from build123d import *

# Parameters (mm, degrees)
F1_W           = 102
F1_H           = 42
F1_W_2         = 98
F1_H_2         = 38
F2_DEPTH       = 72
F3_R           = 8.1966630734
F4_DEPTH       = 25
F6_D           = 3.1
F6_DEPTH       = 20
F6_CSINK_D     = 5.5
F6_CSINK_ANGLE = 90
F6_TIP         = 0.9313339595
F7_W           = 102
F7_H           = 42
F8_DEPTH       = 2
F10_D          = 4
F10_DEPTH      = 20
F10_TIP        = 1.2017212381


with BuildPart() as f2:
    # F1 (on Top) → F2 (new body)
    with BuildSketch(Plane.XY):
        Rectangle(F1_W, F1_H)
        Rectangle(F1_W_2, F1_H_2, mode=Mode.SUBTRACT)
    extrude(amount=F2_DEPTH)

    # F3 (on face) → F4 (cut)
    with BuildSketch(Plane(origin=(0, 0, 0), x_dir=(1, 0, 0), z_dir=(0, 0, -1))):
        Circle(F3_R)
    extrude(amount=-F4_DEPTH, mode=Mode.SUBTRACT)

    # F6
    with Locations(Plane(origin=(-51, 0, 0), x_dir=(0, -1, 0), z_dir=(-1, 0, 0))):
        with Locations((0, 67)):
            CounterSinkHole(F6_D / 2, F6_CSINK_D / 2, depth=F6_DEPTH, counter_sink_angle=F6_CSINK_ANGLE)
            with Locations((0, 0, -(F6_DEPTH + F6_TIP / 2))):  # 118° drill point
                Cone(0, F6_D / 2, F6_TIP, mode=Mode.SUBTRACT)

    # F7 (on Top) → F8 (join)
    with BuildSketch(Plane.XY):
        Rectangle(F7_W, F7_H)
    extrude(amount=F8_DEPTH)

    # F10
    with Locations(Plane(origin=(0, 0, 0), x_dir=(1, 0, 0), z_dir=(0, 0, -1))):
        with Locations((25.5, 10.5), (-25.5, 10.5)):
            Hole(F10_D / 2, depth=F10_DEPTH)
            with Locations((0, 0, -(F10_DEPTH + F10_TIP / 2))):  # 118° drill point
                Cone(0, F10_D / 2, F10_TIP, mode=Mode.SUBTRACT)


solid = f2.part
CAD build for the part. Positions are in the model's coordinates, mm. A direction names the side the tool comes from. Coordinates: 2 decimals unless noted, no trailing zeros. Loops run counter-clockwise (first coordinate to the right, second up) from the corner with the lowest first, then second, coordinate; pieces in that order, holes last. Notation, with made-up numbers: (67.5, 85) - (122.5, 85) arc R5 cw to (122.5, 93) - close; hole circle Ø10 at (61, 32.25). An arc over 180 degrees is marked (long way). Use one line per item in the form item = value. Start each with the question number.
1) Band-saw the part on B-B (x = 25.5). Give the cut face in (y, z).
2) Two-plate mould, pull along Z, no slides. Class faces 1 (the face through (-1, 0, 2)), 2 (the face through (-49.394, -0.202, 68.537)), 3 (the face through (26.974, -11.852, 1.014)): +Z half, -Z half, draft (parallel to the pull), parting line (faces both ways), or undercut.
3) Tool access for faces 4 (the face through (-15, -20, 72)), 5 (the face through (-1, -19, 37)): list every direction of +Z, -Z, +X, -X, +Y, -Y with a clear straight run to the whole face (end or side of a thin tool).
4) Drill centre lines: L1, parallel to X at y = -10.5, z = 0.9; L2, parallel to X at y = -12, z = 7; L3, parallel to Y at x = -49.45, z = 67. Where is each one in solid material? Low to high. Write a range as from..to.
5) Band-saw the part on A-A (y = 0). Give the cut face in (x, z).
6) Band-saw the part on C-C (z = 20). Give the cut face in (x, y).
7) Flat gauge pins, fed straight in: pin 1 (6 mm diameter, centred on x = -30.5, y = -3, fed in from -Z); pin 2 (3 mm diameter, centred on x = -15, y = -8.5, fed in from +Z). Where does each tip first touch, or does it go through?
8) Band-saw the part on D-D (y = -10.5). Give the cut face in (x, z), and give its area (3 significant figures).
Check values:
q1.outline = (-21, 0) - (-12.5, 0) - (-12.5, 2) - (-19, 2) - (-19, 72) - (-21, 72) - close; (-8.5, 0) - (21, 0) - (21, 72) - (19, 72) - (19, 2) - (-8.5, 2) - close
q2.face_1 = +Z half
q2.face_2 = undercut
q2.face_3 = draft
q3.face_4 = +Z, +X, -X, +Y, -Y
q3.face_5 = +Z
q4.L1 = -51..-27.5, -23.5..23.5, 27.5..51
q4.L2 = -51..-49, 49..51
q4.L3 = -21..-1.55, 1.55..21
q5.outline = (-51, 0) - (51, 0) - (51, 72) - (49, 72) - (49, 2) - (-49, 2) - (-49, 65.45) - (-49.8, 65.45) - (-51, 64.25) - close; (-51, 69.75) - (-49.8, 68.55) - (-49, 68.55) - (-49, 72) - (-51, 72) - close
q6.outline = (-51, -21) - (51, -21) - (51, 21) - (-51, 21) - close; hole (-49, -19) - (49, -19) - (49, 19) - (-49, 19) - close
q7.pin_1 = 0
q7.pin_2 = 2
q8.outline = (-51, 0) - (-27.5, 0) - (-27.5, 2) - (-49, 2) - (-49, 72) - (-51, 72) - close; (-23.5, 0) - (23.5, 0) - (23.5, 2) - (-23.5, 2) - close; (27.5, 0) - (51, 0) - (51, 72) - (49, 72) - (49, 2) - (27.5, 2) - close
q8.area = 468 mm2
